Autodesk Fusion 360 part; units mm, degrees
sketch "Sketch1" plane through (0, 0, 0) normal (0, 0, 1) x (1, 0, 0)
  line L0 (0, 0) -> (50, 0)
  line L1 (50, 0) -> (50, 80)
  line L2 (50, 80) -> (0, 80)
  line L3 (0, 80) -> (0, 0)
  line L4 (9, 9) -> (41, 9)
  line L5 (41, 9) -> (41, 71)
  line L6 (41, 71) -> (9, 71)
  line L7 (9, 71) -> (9, 9)
  line L8 (2, 62.5) -> (7, 62.5)
  line L9 (7, 62.5) -> (7, 17.5)
  line L10 (7, 17.5) -> (2, 17.5)
  line L11 (2, 17.5) -> (2, 62.5)
  line L12 (0, 40) -> (2, 40)
  line L13 (25, 71) -> (25, 60)
  line L14 (48, 62.5) -> (43, 62.5)
  line L15 (48, 17.5) -> (48, 62.5)
  line L16 (43, 62.5) -> (43, 17.5)
  line L17 (43, 17.5) -> (48, 17.5)
  dimension "d1" = 50
  dimension "d2" = 80
  dimension "d3" = -9
  dimension "d4" = 45
  dimension "d5" = 90
  dimension "d6" = 2
  dimension "d7" = 5
extrude "Extrude1" add sketch "Sketch1" along normal blind 10
sketch "Sketch2" plane through (0, 0, 0) normal (0, 0, -1) x (1, 0, 0)
  line L0 (2, -17.5) -> (7, -17.5)
  line L1 (7, -17.5) -> (7, -62.5)
  line L2 (7, -62.5) -> (2, -62.5)
  line L3 (2, -62.5) -> (2, -17.5)
  line L4 (43, -17.5) -> (48, -17.5)
  line L5 (48, -17.5) -> (48, -62.5)
  line L6 (48, -62.5) -> (43, -62.5)
  line L7 (43, -62.5) -> (43, -17.5)
  line L8 (9, -71) -> (9, -9)
  line L9 (9, -9) -> (41, -9)
  line L10 (41, -9) -> (41, -71)
  line L11 (41, -71) -> (9, -71)
  line L12 (0, 0) -> (0, -80)
  line L13 (0, -80) -> (50, -80)
  line L14 (50, -80) -> (50, 0)
  line L15 (50, 0) -> (0, 0)
  line L16 (0, 0) -> (50, 0)
  line L17 (50, 0) -> (50, -80)
  line L18 (50, -80) -> (0, -80)
  line L19 (0, -80) -> (0, 0)
extrude "Extrude2" add sketch "Sketch2" along normal blind 2 contours L0 L1 L2 L3 | L4 L5 L6 L7 | L12 L13 L14 L15 L16 L17 L18 L19
sketch "Sketch3" plane through (0, 0, 10) normal (0, 0, 1) x (-1, 0, 0)
  line L0 (-7, -17.5) -> (-2, -17.5)
  line L1 (-2, -17.5) -> (-2, -62.5)
  line L2 (-2, -62.5) -> (-7, -62.5)
  line L3 (-7, -62.5) -> (-7, -17.5)
  line L4 (-9, -9) -> (-9, -71)
  line L5 (-9, -71) -> (-41, -71)
  line L6 (-41, -71) -> (-41, -9)
  line L7 (-41, -9) -> (-9, -9)
  line L8 (-48, -17.5) -> (-43, -17.5)
  line L9 (-43, -17.5) -> (-43, -62.5)
  line L10 (-43, -62.5) -> (-48, -62.5)
  line L11 (-48, -62.5) -> (-48, -17.5)
  line L12 (0, -80) -> (0, 0)
  line L13 (0, 0) -> (-50, 0)
  line L14 (-50, 0) -> (-50, -80)
  line L15 (-50, -80) -> (0, -80)
  line L16 (0, -80) -> (-50, -80)
  line L17 (-50, -80) -> (-50, 0)
  line L18 (-50, 0) -> (0, 0)
  line L19 (0, 0) -> (0, -80)
  line L20 (0, -10.5) -> (-50, -10.5)
  line L21 (-50, -10.5) -> (-50, -69.5)
  line L22 (-50, -69.5) -> (0, -69.5)
  line L23 (0, -69.5) -> (0, -10.5)
  line L24 (-4.5, -17.5) -> (-4.5, -10.5)
  line L25 (-4.5, -62.5) -> (-4.5, -69.5)
  line L26 (-45.5, -62.5) -> (-45.5, -69.5)
  line L27 (-45.5, -17.5) -> (-45.5, -10.5)
  circle A0 centre (-4.5, -14) radius 1
  circle A1 centre (-45.5, -14) radius 1
  circle A2 centre (-45.5, -66) radius 1
  circle A3 centre (-4.5, -66) radius 1
  dimension "d12" = 7
  dimension "d13" = 7
  dimension "d14" = 2
  dimension "d15" = 2
  dimension "d16" = 2
  dimension "d17" = 2
extrude "Extrude3" cut sketch "Sketch3" against normal blind 10 contours L24 A0 | L24 A0 | L25 A3 | L25 A3 | L27 A1 | L27 A1 | L26 A2 | L26 A2
extrude "Extrude4" add sketch "Sketch3" along normal blind 2 contours L4 L6 L7 L12 L13 L14 L17 L18 L19 L20 | L4 L5 L6 L12 L14 L15 L16 L17 L19 L22
sketch "Sketch4" plane through (0, 0, 0) normal (0, -1, 0) x (1, 0, 0)
  line L0 (50, -2) -> (50, 12)
  line L1 (50, 12) -> (0, 12)
  line L2 (0, 12) -> (0, -2)
  line L3 (0, -2) -> (50, -2)
  line L4 (25, 12) -> (25, -2)
  circle A0 centre (25, 5) radius 5
  dimension "d22" = 10
extrude "Extrude5" cut sketch "Sketch4" against normal blind 100 contours L4 A0 | L4 A0
sketch "Sketch5" plane through (0, 0, -2) normal (0, 0, -1) x (1, 0, 0)
  line L0 (41, -9) -> (41, -71)
  line L1 (41, -71) -> (9, -71)
  line L2 (9, -71) -> (9, -9)
  line L3 (9, -9) -> (41, -9)
  line L4 (0, -80) -> (50, -80)
  line L5 (50, -80) -> (50, 0)
  line L6 (50, 0) -> (0, 0)
  line L7 (0, 0) -> (0, -80)
  line L8 (10, -80) -> (40, -80)
  line L9 (50, -70) -> (50, -10)
  line L10 (40, 0) -> (10, 0)
  line L11 (0, -10) -> (0, -70)
  line L12 (39.5, -9) -> (10.5, -9)
  line L13 (9, -10.5) -> (9, -69.5)
  line L14 (10.5, -71) -> (39.5, -71)
  line L15 (41, -69.5) -> (41, -10.5)
  arc A0 (10.5, -9) -> (9, -10.5) centre (10.5, -10.5) ccw
  arc A1 (41, -10.5) -> (39.5, -9) centre (39.5, -10.5) ccw
  arc A2 (9, -69.5) -> (10.5, -71) centre (10.5, -69.5) ccw
  arc A3 (39.5, -71) -> (41, -69.5) centre (39.5, -69.5) ccw
  arc A4 (10, 0) -> (0, -10) centre (10, -10) ccw
  arc A5 (50, -10) -> (40, 0) centre (40, -10) ccw
  arc A6 (0, -70) -> (10, -80) centre (10, -70) ccw
  arc A7 (40, -80) -> (50, -70) centre (40, -70) ccw
  point P0 (20, -71)
  point P1 (9, -10.5)
  point P2 (41, -10.5)
  point P3 (41, -69.5)
  point P4 (9, -69.5)
  dimension "d29" = 10
  dimension "d30" = 10
  dimension "d31" = 10
  dimension "d32" = 10
extrude "Extrude6" cut sketch "Sketch5" against normal blind 100 contours L4 L7 A6 | L4 L5 A7 | L6 L7 A4 | L5 L6 A5
extrude "Extrude7" add sketch "Sketch5" against normal up to surface (14 mm away) contours L0 L3 A1 | L0 L1 A3 | L2 L3 A0 | L1 L2 A2
extrude "Extrude8" add 1 faces at (48, 32.5, 3.3333) along direction (-1, 0, 0) blind 0.5
extrude "Extrude9" add 1 faces at (7, 47.5, 3.3333) along direction (-1, 0, 0) blind 0.5
extrude "Extrude10" add 1 faces at (2, 32.5, 3.3333) along direction (1, 0, 0) blind 0.5
extrude "Extrude11" add 1 faces at (43, 47.5, 3.3333) along direction (1, 0, 0) blind 0.5
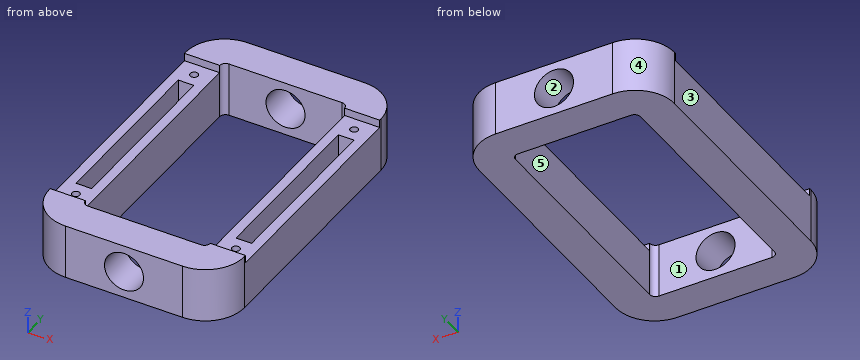
Input: part model. Units: mm. Frame: model coordinates. Face numbers are marked on the shaded views. A direction names the side the tool comes from. Coordinates: 2 decimals unless noted, no trailing zeros. Loops run counter-clockwise (first coordinate to the right, second up) from the corner with the lowest first, then second, coordinate; pieces in that order, holes last. Notation, with made-up numbers: (65, 61.5) -> (124, 61.5) arc R29 cw to (124, 84.5) -> close; hole circle Ø10 at (35.25, -30.5). An arc over 180 degrees is marked (long way). Write each question's results on one line, items separated by ' | '. Start each with the question number.
Q1. Reachability of the marked faces 1 and 2 from +Z, -Z, +X, -X, +Y, -Y: full face, straight path, thin tool, end or side. Return the list, or none.
Q2. Section B-B, the plane x = 25. Return the cut outline in (y, z), plus the area to 3 significant figures.
Q3. Section D-D, the plane z = 9. State how many separate pieces and enclosed holes the cut face has, plus the area to 3 significant figures.
Q4. Pin query (flat end, axial travel): pin 1 (2 mm diameter, centred on x = 45, z = 11, fed in from -Y); pin 2 (1 mm diameter, centred on x = 5, y = 65.5, fed in from +Z); pin 3 (1.5 mm diameter, centred on y = 48, z = 5, fed in from -X); pin 4 (1.6 mm diameter, centred on x = 4.5, z = 11, fed in from +Y). Return the tip coordinate at first contact, or that it passes through.
Q5. Pull-direction query (Y, two-part tool) for the marked faces 3, 4 and 5; classes: released by +Y, released by -Y, zero draft, split by the parting line, or undercut.
Q6. Section A-A, the plane y = 68. Return the cut outline in (x, z), plus the area to 3 significant figures.
Q7. Ray query, line 1 (X direction, y = 14, z = 3.75); line 2 (X direction, y = 39.5, z = 2.5); line 3 (X direction, y = 68, z = 5.75). Return the intervals inside material, ascending. Write a range as from..to.
Q8. Section C-C, the plane x = 12. Return the cut outline in (y, z).
Found:
1) face 1: +Z, -Z | face 2: +Y, -Y
2) outline: (0, -2) -> (9, -2) -> (9, 0) -> (0, 0) -> close; (0, 10) -> (9, 10) -> (9, 12) -> (0, 12) -> close; (71, -2) -> (80, -2) -> (80, 0) -> (71, 0) -> close; (71, 10) -> (80, 10) -> (80, 12) -> (71, 12) -> close | area: 72.0 mm2
3) separate pieces: 2 | enclosed holes: 6 | area: 1,450 mm2
4) pin 1: y = 0.83 | pin 2: z = 10 | pin 3: x = 0 | pin 4: y = 78.83
5) face 3: zero draft | face 4: released by +Y | face 5: undercut
6) outline: (0, -2) -> (9, -2) -> (9, 10) -> (0, 10) -> close; (41, -2) -> (50, -2) -> (50, 10) -> (41, 10) -> close | area: 216 mm2
7) line 1: 0..3.5, 5.5..9, 41..44.5, 46.5..50 | line 2: 0..2.5, 6.5..9, 41..43.5, 47.5..50 | line 3: 0..9, 41..50
8) outline: (0, -2) -> (9, -2) -> (9, 12) -> (0, 12) -> close; (71, -2) -> (80, -2) -> (80, 12) -> (71, 12) -> close
